Here's how the part is built. I have some questions about the finished solid (model axes, mm). Face numbers are marked on the shaded views. Give positions to 0.01 mm unless a question says otherwise; leave off trailing zeros. Order: outer loops, then holes, each group sorted by start corner. A loop starts at its lowest first (then second) coordinate and runs counter-clockwise, first axis right, second up. Notation, with made-up numbers: M -32,-37 L -18,-37 A20 cw -18,-12 Z; hole C 53.25,-6.5 d10. An arc over 180 degrees is marked long. Use one line per item in the form item = value.
from build123d import *

# Parameters (mm, degrees)
SKETCH1_R             = 1.25
BOSS_EXTRUDE1_DEPTH   = 7
BOSS_EXTRUDE2_DEPTH   = 7
BOSS_EXTRUDE2_2_DEPTH = 7
SKETCH1_7_R           = 30
SKETCH1_7_R_2         = 10
BOSS_EXTRUDE3_DEPTH   = 57


with BuildPart() as part:
    # Sketch1 → Boss-Extrude1 (new body)
    with BuildSketch(Plane.XY):
        with BuildLine():
            ThreePointArc((-64.722279519, 146.054710198), (-65.665567973, 148.010892491), (-67.783598849, 148.490879447))
            ThreePointArc((-67.783598849, 148.490879447), (-91.342632394, 140.523795103), (-112.858133693, 128.050395473))
            ThreePointArc((-112.858133693, 128.050395473), (-114.521185483, 127.585787298), (-116.088710674, 128.309988089))
            Line((-116.088710674, 128.309988089), (-126.856076193, 139.077353608))
            ThreePointArc((-126.856076193, 139.077353608), (-127.588245091, 140.863029774), (-126.830567952, 142.638032879))
            ThreePointArc((-126.830567952, 142.638032879), (-39.71763232, 177.992417004), (47.395303312, 142.638032879))
            ThreePointArc((47.395303312, 142.638032879), (48.15298045, 140.863029774), (47.420811552, 139.077353608))
            Line((47.420811552, 139.077353608), (36.653446033, 128.309988089))
            ThreePointArc((36.653446033, 128.309988089), (35.085920842, 127.585787298), (33.422869053, 128.050395473))
            ThreePointArc((33.422869053, 128.050395473), (11.907367753, 140.523795103), (-11.651665791, 148.490879447))
            ThreePointArc((-11.651665791, 148.490879447), (-13.769696668, 148.010892491), (-14.712985122, 146.054710198))
            Line((-14.712985122, 146.054710198), (-14.712985122, 76.440036381))
            ThreePointArc((-14.712985122, 76.440036381), (-16.23263232, 74.140273701), (-18.944111829, 74.636373352))
            ThreePointArc((-18.944111829, 74.636373352), (-39.71763232, 82.992417004), (-60.491152811, 74.636373352))
            ThreePointArc((-60.491152811, 74.636373352), (-63.20263232, 74.140273701), (-64.722279519, 76.440036381))
            Line((-64.722279519, 76.440036381), (-64.722279519, 146.054710198))
        make_face()
        with Locations((-39.71763232, 92.992417004)):
            Circle(SKETCH1_R, mode=Mode.SUBTRACT)
        with Locations((-110.327911654, 143.762392505)):
            Circle(SKETCH1_R, mode=Mode.SUBTRACT)
        with Locations((30.892647013, 143.762392505)):
            Circle(SKETCH1_R, mode=Mode.SUBTRACT)
    extrude(amount=BOSS_EXTRUDE1_DEPTH)



with BuildPart() as body_2:
    # Sketch1_5 → Boss-Extrude2 (new body)
    with BuildSketch(Plane.XY):
        with BuildLine():
            ThreePointArc((-141.289999118, 78.804960004), (-141.334529419, 53.935289488), (-136.454710083, 29.549025778))
            ThreePointArc((-136.454710083, 29.549025778), (-134.980013747, 27.954750711), (-132.81426596, 28.115930093))
            Line((-132.81426596, 28.115930093), (-72.526189959, 62.923267002))
            ThreePointArc((-72.526189959, 62.923267002), (-69.774713456, 62.757095263), (-68.848608602, 60.160835301))
            ThreePointArc((-68.848608602, 60.160835301), (-65.698394434, 37.992417004), (-48.075088111, 24.180042358))
            ThreePointArc((-48.075088111, 24.180042358), (-46.289713456, 22.079882047), (-47.52154276, 19.613947629))
            Line((-47.52154276, 19.613947629), (-107.809618762, -15.19338928))
            ThreePointArc((-107.809618762, -15.19338928), (-109.032078095, -16.988392191), (-108.388743554, -19.062654214))
            ThreePointArc((-108.388743554, -19.062654214), (-89.709529345, -35.481833579), (-68.149497745, -47.878104465))
            ThreePointArc((-68.149497745, -47.878104465), (-66.915609368, -49.086045475), (-66.759023055, -50.805662507))
            Line((-66.759023055, -50.805662507), (-70.700152367, -65.514157338))
            ThreePointArc((-70.700152367, -65.514157338), (-71.88050884, -67.041072287), (-73.79654519, -67.272406189))
            ThreePointArc((-73.79654519, -67.272406189), (-147.970807793, -9.507582996), (-160.909480822, 83.611624322))
            ThreePointArc((-160.909480822, 83.611624322), (-159.751121611, 85.155293524), (-157.838596239, 85.414054741))
            Line((-157.838596239, 85.414054741), (-143.130101408, 81.47292543))
            ThreePointArc((-143.130101408, 81.47292543), (-141.71916253, 80.477509189), (-141.289999118, 78.804960004))
        make_face()
    extrude(amount=BOSS_EXTRUDE2_DEPTH)


with BuildPart() as body_3:
    # Sketch1_5 → Boss-Extrude2 2 (new body)
    with BuildSketch(Plane.XY):
        with BuildLine():
            ThreePointArc((-11.285766896, -47.878104465), (10.274264705, -35.481833579), (28.953478913, -19.062654214))
            ThreePointArc((28.953478913, -19.062654214), (29.596813454, -16.988392191), (28.374354121, -15.19338928))
            Line((28.374354121, -15.19338928), (-31.91372188, 19.613947629))
            ThreePointArc((-31.91372188, 19.613947629), (-33.145551185, 22.079882047), (-31.360176529, 24.180042358))
            ThreePointArc((-31.360176529, 24.180042358), (-13.736870207, 37.992417004), (-10.586656039, 60.160835301))
            ThreePointArc((-10.586656039, 60.160835301), (-9.660551185, 62.757095263), (-6.909074682, 62.923267002))
            Line((-6.909074682, 62.923267002), (53.37900132, 28.115930093))
            ThreePointArc((53.37900132, 28.115930093), (55.544749107, 27.954750711), (57.019445442, 29.549025778))
            ThreePointArc((57.019445442, 29.549025778), (61.899264778, 53.935289488), (61.854734477, 78.804960004))
            ThreePointArc((61.854734477, 78.804960004), (62.28389789, 80.477509189), (63.694836768, 81.47292543))
            Line((63.694836768, 81.47292543), (78.403331598, 85.414054741))
            ThreePointArc((78.403331598, 85.414054741), (80.31585697, 85.155293524), (81.474216181, 83.611624322))
            ThreePointArc((81.474216181, 83.611624322), (68.535543153, -9.507582996), (-5.638719451, -67.272406189))
            ThreePointArc((-5.638719451, -67.272406189), (-7.5547558, -67.041072287), (-8.735112274, -65.514157338))
            Line((-8.735112274, -65.514157338), (-12.676241586, -50.805662507))
            ThreePointArc((-12.676241586, -50.805662507), (-12.519655272, -49.086045475), (-11.285766896, -47.878104465))
        make_face()
    extrude(amount=BOSS_EXTRUDE2_2_DEPTH)


with BuildPart() as part_1:
    add(part.part)

    add(body_2.part)  # Boss-Extrude3 merges body 2

    add(body_3.part)  # Boss-Extrude3 merges body 3
    # Sketch1_7 → Boss-Extrude3 (add)
    with BuildSketch(Plane.XY):
        with Locations(Location((-39.71763232, 52.992417004, 0), (0, 0, 166.175583888))):
            Circle(SKETCH1_7_R)
        with Locations(Location((-39.71763232, 52.992417004, 0), (0, 0, 180))):
            Circle(SKETCH1_7_R_2, mode=Mode.SUBTRACT)
    extrude(amount=BOSS_EXTRUDE3_DEPTH)


solid = part_1.part
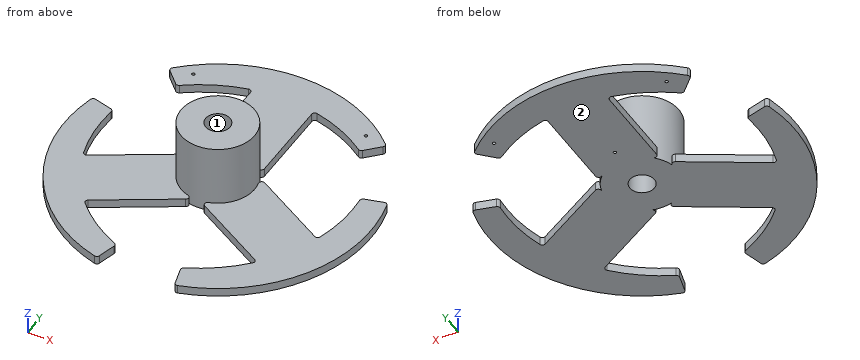
Q1. I need wall thicknesses on L1, parallel to X at y = 52.5, z = 23.5; L2, parallel to Z at x = 58, y = 31.5; L3, parallel to Y at x = -71, z = 4.5. Which ranges of each line are inside material? Lowest first, please.
Found:
L1 = -69.71 to -49.71, -29.73 to -9.72
L2 = 0 to 7
L3 = -66.2 to -46.55, 6.06 to 63.24, 147.7 to 174.01
Q2. I want a section at C-C on x = 3. Write out the boundary of the cut face in (y, z), then the cut area to 3 significant figures.
Found:
outline = M -64.48,0 L -40.32,0 L -40.32,7 L -64.48,7 Z; M -0.54,0 L 57.2,0 L 57.2,7 L -0.54,7 Z; M 144.16,0 L 170.47,0 L 170.47,7 L 144.16,7 Z
area = 758 mm²
Q3. Thinking about a two-plate mould opening in X: for the marked faces 1 and 2, which applies, +X half, -X half, draft (parallel to the pull), parting line (faces both ways), or undercut?
Found:
face_1 = undercut
face_2 = draft
Q4. I'm going to push flat-ended pins straight in: pin 1 Ø1.5 at (y, z) = (64, 45.5) entering from -X; pin 2 Ø10 at (x, z) = (-52, 46) entering from -Y; pin 3 Ø2 at (x, y) = (-110.33, 143.76) entering from -Z; pin 4 Ø12 at (x, y) = (-78.5, -4.5) entering from +Z. Where does each tip first touch, or does it pass through?
Found:
pin_1 = -67.91
pin_2 = 23.89
pin_3 = through
pin_4 = 7
Q5. I want a section at A-A on y = 35. Write out the boundary of the cut face in (x, z).
Found:
outline = M -163.42,0 L -137.99,0 L -137.99,7 L -163.42,7 Z; M -120.89,0 L 41.46,0 L 41.46,7 L -15.71,7 L -15.71,57 L -63.72,57 L -63.72,7 L -120.89,7 Z; M 58.55,0 L 83.98,0 L 83.98,7 L 58.55,7 Z
Q6. I want a section at D-D on z = 27.5. Write out the boundary of the cut face in (x, y).
Found:
outline = C -39.72,52.99 d60; hole C -39.72,52.99 d20
Q7. I want a section at B-B on y = -8. Write out the boundary of the cut face in (x, z).
Found:
outline = M -148.83,0 L -95.35,0 L -95.35,7 L -148.83,7 Z; M 15.92,0 L 69.39,0 L 69.39,7 L 15.92,7 Z
